Input: part model. Units: mm. Frame: model coordinates. Face numbers are marked on the shaded views. A direction names the side the tool comes from. Give positions to 0.01 mm unless a question says otherwise; leave off trailing zeros. Order: outer loops, then holes, each group sorted by start corner. A loop starts at its lowest first (then second) coordinate and runs counter-clockwise, first axis right, second up.
Autodesk Inventor part; units mm, degrees
ref_plane "YZ Plane" through (0, 0, 0) normal (1, 0, 0) x (0, 1, 0)
ref_plane "XZ Plane" through (0, 0, 0) normal (0, 1, 0) x (-1, 0, 0)
ref_plane "XY Plane" through (0, 0, 0) normal (0, 0, 1) x (1, 0, 0)
sketch "Sketch1" plane through (0, 0, 0) normal (1, 0, 0) x (0, 1, 0)
  line L0 (4.4986, 14.2657) -> (-15.5014, 14.2657)
  line L1 (-15.5014, 14.2657) -> (-15.5014, -15.7343)
  line L2 (-15.5014, -15.7343) -> (4.4986, -15.7343)
  line L3 (4.4986, -15.7343) -> (4.4986, 14.2657)
  point P0 (0, 0)
  dimension "d0" = 20
  dimension "d1" = 30
extrude "Extrusion1" add sketch "Sketch1" along normal blind 20
sketch "Sketch2" plane through (20, 0, 0) normal (1, 0, 0) x (0, 0, -1)
  line L0 (-13.0153, 3.3051) -> (14.6165, 3.3051)
  line L1 (14.6165, 3.3051) -> (14.6165, -14.4728)
  line L2 (14.6165, -14.4728) -> (-13.0153, -14.4728)
  line L3 (-13.0153, -14.4728) -> (-13.0153, 3.3051)
  point P0 (0, 0)
extrude "Extrusion2" cut sketch "Sketch2" against normal blind 18
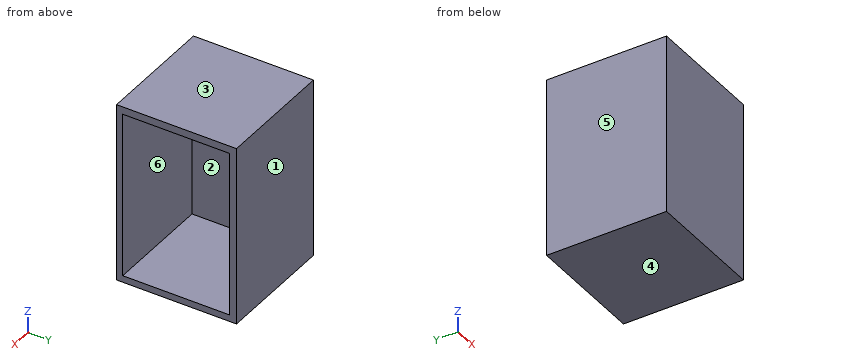
1) Cut plane C-C (y = -10.25). Return the cut outline in (x, z), then the cut area to 3 significant figures.
2) First-contact query: P1, Ø9, axis at y = -4.5, z = 1.5, coming from the +X side. Flat tip, straight axial feed; report the tip coordinate or a pass-through.
3) Pull-direction query (Z, two-part tool) for the marked faces 3, 4, 5 and 6; classes: pulls with the +Z half, pulls with the -Z half, needs draft (parallel to the pull), parting line crosses it, or undercut.
4) Cut plane A-A (x = 8.5). Return the cut outline in (y, z).
5) Cut plane B-B (z = -1). Return the cut outline in (x, y).
6) Reachability of the marked faces 1 and 2 from +Z, -Z, +X, -X, +Y, -Y: full face, straight path, thin tool, end or side. Return the list, or none.
7) Line query: probe 1 along Z at (x, y) = (6, 3.25); probe 2 along Y at (x, z) = (18, -9.5); probe 3 along X at (y, z) = (0.5, -6). Output: solid intervals per line, ascending.
Geometry says:
1. outline: (0, -15.73) - (20, -15.73) - (20, -14.62) - (2, -14.62) - (2, 13.02) - (20, 13.02) - (20, 14.27) - (0, 14.27) - close
1. area: 103 mm2
2. P1: stops at x = 2
3. face 3: pulls with the +Z half
3. face 4: pulls with the -Z half
3. face 5: needs draft
3. face 6: undercut
4. outline: (-15.5, -15.73) - (4.5, -15.73) - (4.5, 14.27) - (-15.5, 14.27) - close; hole (-14.47, -14.62) - (3.31, -14.62) - (3.31, 13.02) - (-14.47, 13.02) - close
5. outline: (0, -15.5) - (20, -15.5) - (20, -14.47) - (2, -14.47) - (2, 3.31) - (20, 3.31) - (20, 4.5) - (0, 4.5) - close
6. face 1: +Z, -Z, +X, -X, +Y
6. face 2: +X
7. probe 1: z = -15.73 to -14.62, 13.02 to 14.27
7. probe 2: y = -15.5 to -14.47, 3.31 to 4.5
7. probe 3: x = 0 to 2
